```python
from build123d import *

# Parameters (mm, degrees)
BOSS_EXTRUDE1_DEPTH      = 6.86
SKETCH2_R                = 5
SKETCH2_R_2              = 16
CUT_EXTRUDE1_DEPTH       = 6.86
SKETCH3_W                = 11.5
SKETCH3_H                = 19
SKETCH3_W_2              = 7
BOSS_EXTRUDE2_DEPTH      = 5.5
SKETCH4_R                = 1.165
CUT_EXTRUDE2_DEPTH       = 12.5
SKETCH6_R                = 12
CUT_EXTRUDE3_DEPTH       = 1
SKETCH7_R                = 1.5
SKETCH7_R_2              = 1.493707415
BOSS_EXTRUDE5_DEPTH      = 1
BOSS_EXTRUDE5_DEPTH_BACK = 1


with BuildPart() as part:
    # Sketch1 → Boss-Extrude1 (new body)
    with BuildSketch(Plane(origin=(0, 0, 0), x_dir=(1, 0, 0), z_dir=(0, 1, 0))):
        with BuildLine():
            Line((-13.264052164, 25), (36.735947836, 25))
            ThreePointArc((36.735947836, 25), (61.735947836, 0), (36.735947836, -25))
            Line((36.735947836, -25), (-13.264052164, -25))
            ThreePointArc((-13.264052164, -25), (-38.264052164, 0), (-13.264052164, 25))
        make_face()
    extrude(amount=BOSS_EXTRUDE1_DEPTH)

    # Sketch2 → Cut-Extrude1 (cut)
    with BuildSketch(Plane(origin=(0, 6.86, 0), x_dir=(1, 0, 0), z_dir=(0, 1, 0))):
        with Locations((36.735947836, 0)):
            Circle(SKETCH2_R)
        with Locations((-13.264052164, 0)):
            Circle(SKETCH2_R_2)
    extrude(amount=-CUT_EXTRUDE1_DEPTH, mode=Mode.SUBTRACT)

    # Sketch3 → Boss-Extrude2 (add)
    with BuildSketch(Plane.XZ):
        with Locations((-27.554052164, -0.231081814)):
            Rectangle(SKETCH3_W, SKETCH3_H)
        with Locations((18.195874459, -0.141240273)):
            Rectangle(SKETCH3_W_2, SKETCH3_H)
    extrude(amount=BOSS_EXTRUDE2_DEPTH)

    # Sketch4 → Cut-Extrude2 (cut)
    with BuildSketch(Plane.XZ.offset(5.5)):
        with Locations((-23.104052164, 4.678918186)):
            Circle(SKETCH4_R)
        with Locations((-23.104052164, -5.211081814)):
            Circle(SKETCH4_R)
    extrude(amount=-CUT_EXTRUDE2_DEPTH, mode=Mode.SUBTRACT)

    # Sketch6 → Cut-Extrude3 (cut)
    with BuildSketch(Plane(origin=(0, 0, 0), x_dir=(1, 0, 0), z_dir=(0, 1, 0))):
        with Locations((36.735947836, 0)):
            Circle(SKETCH6_R)
    extrude(amount=CUT_EXTRUDE3_DEPTH, mode=Mode.SUBTRACT)

    # Sketch7 → Boss-Extrude5 (add, two sides)
    with BuildSketch(Plane(origin=(0, 0, 0), x_dir=(1, 0, 0), z_dir=(0, 1, 0))) as boss_extrude5_sk:
        with Locations((36.735947836, -9)):
            Circle(SKETCH7_R)
        with Locations((29.268034032, 5.059173887)):
            Circle(SKETCH7_R_2)
        with Locations((44.243842587, 4.965825904)):
            Circle(SKETCH7_R)
    extrude(amount=BOSS_EXTRUDE5_DEPTH)
    extrude(boss_extrude5_sk.sketch, amount=-BOSS_EXTRUDE5_DEPTH_BACK)


solid = part.part
```
Design review of the part built by this model. Coordinates are the model's own, in mm. A direction names the side the tool comes from. Coordinates: 2 decimals unless noted, no trailing zeros. Order: outer loops, then holes, each group sorted by start corner. A loop starts at its lowest first (then second) coordinate and runs counter-clockwise, first axis right, second up.
1) Take a section at D-D, the plane z = -8.5. Give the boundary of the cut face in (x, y), and give its area (3 significant figures).
2) For faces 5 (the flat face through (18, -3, -9.641)), 6 (the flat face through (-33.304, -3, 0)), 7 (the flat face through (36.6, 1, 5.2)), list the 3-axis set-ups (+Z, -Z, +X, -X, +Y, -Y) from which the entire face can be reached by the end or side of a thin tool; tool diameter is ignored.
3) Clearance check with flat-ended pins moving along their axes: pin 1 (4.5 mm diameter, centred on x = 19, y = -1.5, fed in from -Z); pin 2 (1.4 mm diameter, centred on x = -23.1, z = -5.21, fed in from +Y); pin 3 (6 mm diameter, centred on x = 34, z = -13, fed in from -Y); pin 4 (6 mm diameter, centred on x = -26, y = -4, fed in from +Z). State where each tip first meets the part, or that it passes through.
4) Wall thickness on line 1 along X through (y, z) = (5.25, 0); line 2 along Y through (x, z) = (-25, 2); line 3 along Y through (x, z) = (12, 21): over which ranges is each line inside the solid? List them lowest first.
5) Mouldability with a two-part tool opening along X and no side actions: class faces 1 (the flat face through (14.696, -3, 0)), 2 (the cylindrical face through (-38.26, 3.38, 0.55)), 3 (the cylindrical face through (-22.03, -2.79, 4.23)), 4 (the flat face through (-28, -5.5, 0)) as +X half, -X half, draft (parallel to the pull), parting line (faces both ways), or undercut.
6) Take a section at B-B, the plane y = 3.5. Give the boundary of the cut face in (x, z), and give its area (3 significant figures).
7) Take a section at A-A, the plane z = 0. Give the boundary of the cut face in (x, y), and give its area (3 significant figures).
8) Take a section at C-C, the plane x = -4. Give the boundary of the cut face in (y, z), and give its area (3 significant figures).
Returned:
1. outline: (-36.77, 0) - (-33.3, 0) - (-33.3, -5.5) - (-21.8, -5.5) - (-21.8, 0) - (-26.82, 0) - (-26.82, 6.86) - (-36.77, 6.86) - close; (0.29, 0) - (14.7, 0) - (14.7, -5.5) - (21.7, -5.5) - (21.7, 0) - (28.27, 0) - (28.27, 1) - (45.21, 1) - (45.21, 0) - (60.25, 0) - (60.25, 6.86) - (0.29, 6.86) - close
1. area: 564 mm2
2. face 5: -Z, +X, -Y
2. face 6: +Z, -Z, -X, -Y
2. face 7: -Y
3. pin 1: stops at z = -25
3. pin 2: passes through
3. pin 3: stops at y = 0
3. pin 4: stops at z = 9.27
4. line 1: x = -38.26 to -29.26, 2.74 to 31.74, 41.74 to 61.74
4. line 2: y = -5.5 to 0
4. line 3: y = 0 to 6.86
5. face 1: undercut
5. face 2: -X half
5. face 3: undercut
5. face 4: draft
6. outline: (-13.26, -25) - (36.74, -25) arc R25 ccw to (36.74, 25) - (-13.26, 25) arc R25 ccw to start; hole circle Ø32 at (-13.26, 0); hole circle Ø10 at (36.74, 0)
6. area: 3,580 mm2
7. outline: (-38.26, 0) - (-33.3, 0) - (-33.3, -5.5) - (-21.8, -5.5) - (-21.8, 0) - (-29.26, 0) - (-29.26, 6.86) - (-38.26, 6.86) - close; (2.74, 0) - (14.7, 0) - (14.7, -5.5) - (21.7, -5.5) - (21.7, 0) - (24.74, 0) - (24.74, 1) - (31.74, 1) - (31.74, 6.86) - (2.74, 6.86) - close; (41.74, 1) - (48.74, 1) - (48.74, 0) - (61.74, 0) - (61.74, 6.86) - (41.74, 6.86) - close
7. area: 486 mm2
8. outline: (0, -25) - (6.86, -25) - (6.86, -13.05) - (0, -13.05) - close; (0, 13.05) - (6.86, 13.05) - (6.86, 25) - (0, 25) - close
8. area: 164 mm2
